Can you work these out from the model? Positions are in its coordinate system, mm. A direction names the side the tool comes from. Give positions to 0.01 mm unless a question says otherwise; leave off trailing zeros. Write each loop counter-clockwise with the first axis right and the second up, starting at its lowest first coordinate (ties: lowest second). Pieces come first, ordered by that corner, then holes. Notation, with made-up numbers: M 70,13.25 L 102,13.25 A14 ccw 102,27.25 Z; hole C -26.75,27 d3. An arc over 180 degrees is marked long. Write each question's results on one line, items separated by ' | '.
from build123d import *

# Parameters (mm, degrees)
F1_DEPTH = 9.525
F2_R     = 10.16


with BuildPart() as f1:
    # F0 (on Front) → F1 (new body)
    with BuildSketch(Plane.XZ):
        Polygon((-31.945355, 53.413631), (-57.344088, 53.159991), (-57.344088, -73.840009), (37.905912, -73.840009), (37.905912, -48.440009), align=None)
        Polygon((-38.294088, -54.790009), (-38.294088, 28.988602), (19.161316, -54.790009), align=None, mode=Mode.SUBTRACT)
    extrude(amount=F1_DEPTH)

    # F2
    f2_edges = [f1.edges().sort_by_distance(p)[0] for p in [
        (-38.294088, -4.7625, -54.790009),
        (19.161316, -4.7625, -54.790009),
        (-38.294088, -4.7625, 28.988602),
    ]]
    fillet(f2_edges, radius=F2_R)


solid = f1.part
Item 1: I want a section at D-D, the plane z = 35. Please give me the cut outline in (x, y) (3 decimals), and give its area (3 significant figures).
Geometry says:
outline: M -57.344,-9.525 L -19.317,-9.525 L -19.317,0 L -57.344,0 Z | area: 362 mm2
Item 2: I'm going to push a flat-ended pin straight in: pin 1 (5 mm diameter, centred on y = -4.5, z = -17.5, fed in from +X). Where does the tip first touch, or does it pass through?
Geometry says:
pin 1: stops at x = 18.4
Item 3: For faces 4 (the face through (-14, -5, -54.79)), 5 (the face through (-57.344, -5, -9)), which set-ups out of +Z, -Z, +X, -X, +Y, -Y let a thin tool reach every point of the face, with its end or its side?
Geometry says:
face 4: +Y, -Y | face 5: +Z, -Z, -X, +Y, -Y
Item 4: I want a section at A-A, the plane y = -4. Please give me the cut outline in (x, z).
Geometry says:
outline: M -57.34,-73.84 L 37.91,-73.84 L 37.91,-48.44 L -31.95,53.41 L -57.34,53.16 Z; hole M -38.29,-44.63 A10.16 ccw -28.13,-54.79 L -0.13,-54.79 A10.16 ccw 8.25,-38.88 L -19.76,1.96 A10.16 ccw -38.29,-3.79 Z
Item 5: Thinking about a two-plate mould opening in X: for faces 1 (the face through (37.906, -5, -61)), 2 (the face through (-5.947, -4.696, -18.178)), 3 (the face through (-10, -9.525, -9)), which applies, +X half, -X half, draft (parallel to the pull), parting line (faces both ways), or undercut?
Geometry says:
face 1: +X half | face 2: undercut | face 3: draft
Item 6: If I drill on line 1 (X direction, y = -5.75, z = -7.5); line 2 (X direction, y = -2.75, z = -38); line 3 (Z direction, x = -19.5, y = -4), over which ranges is the centre line in solid material (lowest first)? Write a range as from..to.
Geometry says:
line 1: x = -57.34..-38.29, -13.27..9.83 | line 2: x = -57.34..-38.29, 7.65..30.75 | line 3: z = -73.84..-54.79, 1.58..35.27
Item 7: I want a section at B-B, the plane z = -24. Please give me the cut outline in (x, y) (3 decimals).
Geometry says:
outline: M -57.344,-9.525 L -38.294,-9.525 L -38.294,0 L -57.344,0 Z; M -1.954,-9.525 L 21.145,-9.525 L 21.145,0 L -1.954,0 Z
Item 8: I want a section at C-C, the plane x = -8. Please give me the cut outline in (y, z) (3 decimals).
Geometry says:
outline: M -9.525,-73.84 L 0,-73.84 L 0,-54.79 L -9.525,-54.79 Z; M -9.525,-15.185 L 0,-15.185 L 0,18.498 L -9.525,18.498 Z
